Input: part model. Units: mm. Frame: model coordinates. Face numbers are marked on the shaded views. Coordinates: 2 decimals unless noted, no trailing zeros. Loops run counter-clockwise (first coordinate to the right, second up) from the corner with the lowest first, then second, coordinate; pieces in that order, holes last.
```python
from build123d import *

# Parameters (mm, degrees)
BOSS_EXTRUDE1_DEPTH             = 227.5
TAP_DRILL_FOR_M5X0_8_TAP1_D     = 5
TAP_DRILL_FOR_M5X0_8_TAP1_DEPTH = 10
TAP_DRILL_FOR_M5X0_8_TAP2_D     = 5
TAP_DRILL_FOR_M5X0_8_TAP2_DEPTH = 10
TAP_DRILL_FOR_M5X0_8_TAP3_D     = 5
TAP_DRILL_FOR_M5X0_8_TAP3_DEPTH = 10
TAP_DRILL_FOR_M5X0_8_TAP4_D     = 5
TAP_DRILL_FOR_M5X0_8_TAP4_DEPTH = 10
SKETCH11_R                      = 1.5
CUT_EXTRUDE1_DEPTH              = 29
SKETCH13_R                      = 1.5
CUT_EXTRUDE2_DEPTH              = 29


with BuildPart() as part:
    # Sketch1 → Boss-Extrude1 (new body)
    with BuildSketch(Plane.XY):
        Polygon((44.5, 5.5), (-44.5, 5.5), (-44.5, 14.835), (-50.17, 14.835), (-50.17, 20.5), (-59.5, 20.5), (-59.5, 0), (59.5, 0), (59.5, 20.5), (50.17, 20.5), (50.17, 14.835), (44.5, 14.835), align=None)
    extrude(amount=BOSS_EXTRUDE1_DEPTH)

    # Tap Drill for M5x0.8 Tap1
    with Locations(Plane.XY.offset(227.5)):
        with Locations((52, 8), (-52, 8)):
            Hole(TAP_DRILL_FOR_M5X0_8_TAP1_D / 2, depth=TAP_DRILL_FOR_M5X0_8_TAP1_DEPTH)

    # Tap Drill for M5x0.8 Tap2
    with Locations(Plane(origin=(0, 0, 0), x_dir=(-1, 0, 0), z_dir=(0, 0, -1))):
        with Locations((52, 8), (-52, 8)):
            Hole(TAP_DRILL_FOR_M5X0_8_TAP2_D / 2, depth=TAP_DRILL_FOR_M5X0_8_TAP2_DEPTH)

    # Tap Drill for M5x0.8 Tap3
    with Locations(Plane(origin=(59.5, 0, 0), x_dir=(0, 0, -1), z_dir=(1, 0, 0))):
        with Locations((-193.75, 10), (-153.75, 10), (-113.75, 10), (-73.75, 10), (-33.75, 10)):
            Hole(TAP_DRILL_FOR_M5X0_8_TAP3_D / 2, depth=TAP_DRILL_FOR_M5X0_8_TAP3_DEPTH)

    # Tap Drill for M5x0.8 Tap4
    with Locations(Plane.ZY.offset(59.5)):
        with Locations((193.75, 10), (153.75, 10), (113.75, 10), (73.75, 10), (33.75, 10)):
            Hole(TAP_DRILL_FOR_M5X0_8_TAP4_D / 2, depth=TAP_DRILL_FOR_M5X0_8_TAP4_DEPTH)

    # Sketch11 → Cut-Extrude1 (cut)
    with BuildSketch(Plane.XZ):
        with Locations((-47.33, 173.75)):
            Circle(SKETCH11_R)
        with Locations((-47.33, 133.75)):
            Circle(SKETCH11_R)
        with Locations((-47.33, 93.75)):
            Circle(SKETCH11_R)
        with Locations((-47.33, 53.75)):
            Circle(SKETCH11_R)
        with Locations(Location((47.33, 53.75, 0), (0, 0, 270))):
            Circle(SKETCH11_R)
        with Locations(Location((47.33, 93.75, 0), (0, 0, 270))):
            Circle(SKETCH11_R)
        with Locations(Location((47.33, 133.75, 0), (0, 0, 270))):
            Circle(SKETCH11_R)
        with Locations(Location((47.33, 173.75, 0), (0, 0, 270))):
            Circle(SKETCH11_R)
    extrude(amount=-CUT_EXTRUDE1_DEPTH, mode=Mode.SUBTRACT)

    # Sketch13 → Cut-Extrude2 (cut)
    with BuildSketch(Plane.ZY.offset(-50.17)):
        with Locations((193.75, 17.6675)):
            Circle(SKETCH13_R)
        with Locations((153.75, 17.6675)):
            Circle(SKETCH13_R)
        with Locations((113.75, 17.6675)):
            Circle(SKETCH13_R)
        with Locations((73.75, 17.6675)):
            Circle(SKETCH13_R)
        with Locations((33.75, 17.6675)):
            Circle(SKETCH13_R)
    extrude(amount=-CUT_EXTRUDE2_DEPTH, mode=Mode.SUBTRACT)


solid = part.part
```
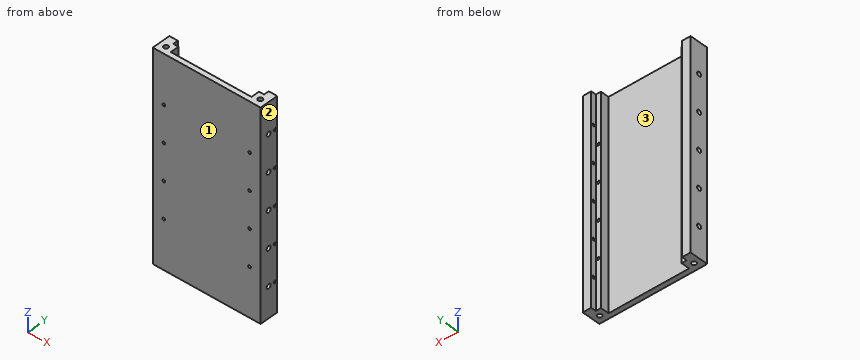
Item 1: Mould query, pull axis X, two halves, no side actions, for the marked faces 1, 2 and 3. Classes: +X half, -X half, draft (parallel to the pull), parting line (faces both ways), or undercut.
Result:
face 1: draft
face 2: +X half
face 3: undercut
Item 2: Line query: L1, parallel to Y at x = 54.5, z = 33.75; L2, parallel to Y at x = 52, z = 6.25; L3, parallel to Z at x = -47.5, y = 14.25. Output: solid intervals per line, ascending.
Result:
L1: y = 0 to 7.5, 12.5 to 16.17, 19.17 to 20.5
L2: y = 0 to 5.5, 10.5 to 20.5
L3: z = 0 to 52.26, 55.24 to 92.26, 95.24 to 132.26, 135.24 to 172.26, 175.24 to 227.5
Item 3: Contact query for flat-ended pins moving along their axis: P1, Ø1.5, axis at x = -53, y = 8.5, coming from the +Z side; P2, Ø1, axis at x = 25.5, z = 84.5, coming from the +Y side; P3, Ø3.5, axis at x = -47.33, z = 133.75, coming from the +Y side (3 decimals). Output: stop coordinate, or through.
Result:
P1: stops at z = 217.5
P2: stops at y = 5.5
P3: stops at y = 14.835
Item 4: Section query A-A (z = 81). Output: boundary loops of the cut face in (x, y) (3 decimals), then the cut area to 3 significant figures.
Result:
outline: (-59.5, 0) - (59.5, 0) - (59.5, 20.5) - (50.17, 20.5) - (50.17, 14.835) - (44.5, 14.835) - (44.5, 5.5) - (-44.5, 5.5) - (-44.5, 14.835) - (-50.17, 14.835) - (-50.17, 20.5) - (-59.5, 20.5) - close
area: 1,040 mm2
Item 5: Section query B-B (x = -24.5). Output: boundary loops of the cut face in (y, z).
Result:
outline: (0, 0) - (5.5, 0) - (5.5, 227.5) - (0, 227.5) - close
